Can you work these out from the drawing? Everything is in mm from the part's minimum corner. Coordinates: 2 decimals unless noted, no trailing zeros. Write each loop counter-clockwise with the first axis right and the second up, starting at its lowest first coordinate (ties: lowest second). Pieces come first, ordered by that corner, then holes.
(1) Imagine slicing it at A-A, the plane x = 44.75. List the corners of the cut face in (y, z) for me, plus the area to 3 significant figures.
(2) For pin 1 Ø1.9 at (x, z) = (11.25, 27.3) entering from -Y, with a flat end and sliding along its axis, tell me the tip position at first contact or that it passes through.
(3) Imagine slicing it at C-C, the plane x = 11.5. List the corners of the cut face in (y, z) for me, plus the area to 3 significant figures.
(4) Imagine slicing it at B-B, the plane y = 1.35. List the corners of the cut face in (x, z) for me.
(5) Please list where these lines run through material, in increasing order: probe 1 along Z at (x, y) = (4.75, 0.9); probe 2 along Z at (x, y) = (38.25, 1.3); probe 3 along Z at (x, y) = (43.5, 1.1).
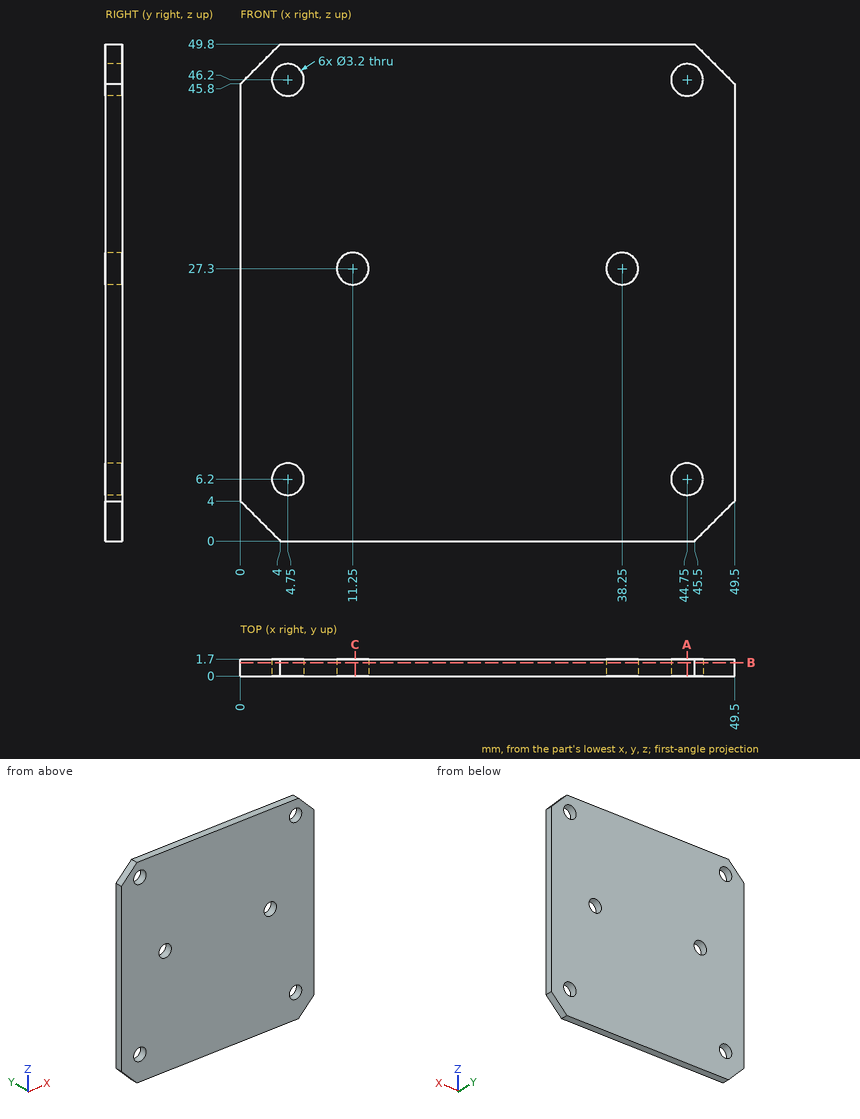
Recorded:
1. outline: (0, 0) - (1.7, 0) - (1.7, 4.6) - (0, 4.6) - close; (0, 7.8) - (1.7, 7.8) - (1.7, 44.6) - (0, 44.6) - close; (0, 47.8) - (1.7, 47.8) - (1.7, 49.8) - (0, 49.8) - close
1. area: 73.8 mm2
2. pin 1: passes through
3. outline: (0, 0) - (1.7, 0) - (1.7, 25.72) - (0, 25.72) - close; (0, 28.88) - (1.7, 28.88) - (1.7, 49.8) - (0, 49.8) - close
3. area: 79.3 mm2
4. outline: (0, 4) - (4, 0) - (45.5, 0) - (49.5, 4) - (49.5, 45.8) - (45.5, 49.8) - (4, 49.8) - (0, 45.8) - close; hole circle Ø3.2 at (4.75, 6.2); hole circle Ø3.2 at (4.75, 46.2); hole circle Ø3.2 at (11.25, 27.3); hole circle Ø3.2 at (38.25, 27.3); hole circle Ø3.2 at (44.75, 6.2); hole circle Ø3.2 at (44.75, 46.2)
5. probe 1: z = 0 to 4.6, 7.8 to 44.6, 47.8 to 49.8
5. probe 2: z = 0 to 25.7, 28.9 to 49.8
5. probe 3: z = 0 to 5.2, 7.2 to 45.2, 47.2 to 49.8
